Geometry: final body of the model. Coordinates: model frame, mm. A direction names the side the tool comes from. Round coordinates to 2 decimals unless told otherwise and drop trailing zeros. Loops run counter-clockwise (first coordinate to the right, second up) from the corner with the lowest first, then second, coordinate; pieces in that order, holes last. Notation, with made-up numbers: (21.25, -13) - (64.25, -13) arc R22 ccw to (64.25, -3) - close; hole circle Ø1 at (87, -1.5). An arc over 180 degrees is marked (long way). Return JSON: item names as keys, results as strings. Group by question number.
1. Draft query along Z for faces 6 (the face through (1.97, -17.85, -11.57)), 7 (the face through (2, -10, -5)), 8 (the face through (2, -20.5, -7)). Return one class per face: +Z half, -Z half, draft (parallel to the pull), parting line (faces both ways), or undercut.
2. Section B-B on x = 3.2. Return loops of the section in (y, z).
3. First-contact query: pin 1 Ø0.8 at (x, y) = (0.5, -2.5) entering from +Z; pin 2 Ø1 at (x, z) = (3, -10) entering from +Y; pin 3 Ø6 at (y, z) = (-8, -1.5) entering from +X; pin 4 Ø0.8 at (x, y) = (1, -6.5) entering from -Z. Flat tips, straight axial feed; report the tip coordinate or a pass-through.
4. Section D-D on y = -6.5. Return loops of the section in (x, z).
5. Section C-C on z = -7.5. Return loops of the section in (x, y).
6. Material intervals for probe 1 along Y at (x, z) = (2.85, -9.75); probe 2 along Y at (x, z) = (3, -5.5); probe 3 along X at (y, z) = (-2, -3.5), sorted ascending.
7. Section A-A on z = -10.25. Return loops of the section in (x, y), and give its area (3 significant figures).
8. Set-up query: faces 1 (the face through (1, -5, -10)), 2 (the face through (2, -19.2, -3.7)), 3 (the face through (2, -20.1, -10)), 4 (the face through (1, -5, 0)), 5 (the face through (1.6, -5, -5)). Return all of +Z, -Z, +X, -X, +Y, -Y with unobstructed straight access to the full face (end or side cutting, diameter ignored); none if empty.
from build123d import *

# Parameters (mm, degrees)
SKETCH1_W           = 10
SKETCH1_H           = 10
BOSS_EXTRUDE1_DEPTH = 1.6
BOSS_EXTRUDE2_DEPTH = 10
SKETCH3_W           = 4
SKETCH3_H           = 2
BOSS_EXTRUDE3_DEPTH = 2
SKETCH4_W           = 4
SKETCH4_H           = 2
BOSS_EXTRUDE4_DEPTH = 2
BOSS_EXTRUDE5_DEPTH = 4
FILLET2_R           = 1.5


with BuildPart() as part:
    # Sketch1 → Boss-Extrude1 (new body)
    with BuildSketch(Plane(origin=(0, 0, 0), x_dir=(0, 0, -1), z_dir=(1, 0, 0))):
        with Locations((5, -5)):
            Rectangle(SKETCH1_W, SKETCH1_H)
    extrude(amount=BOSS_EXTRUDE1_DEPTH)

    # Sketch2 → Boss-Extrude2 (add)
    with BuildSketch(Plane.XY):
        Polygon((1.2, -12), (0, -12), (0, -10), (1.6, -10), (4, -10), (4, -12), (2.8, -12), align=None)
    extrude(amount=-BOSS_EXTRUDE2_DEPTH)

    # Sketch3 → Boss-Extrude3 (add)
    with BuildSketch(Plane.XY):
        with Locations((2, -11)):
            Rectangle(SKETCH3_W, SKETCH3_H)
    extrude(amount=BOSS_EXTRUDE3_DEPTH)

    # Sketch4 → Boss-Extrude4 (add)
    with BuildSketch(Plane(origin=(0, 0, -10), x_dir=(-1, 0, 0), z_dir=(0, 0, -1))):
        with Locations((-2, -11)):
            Rectangle(SKETCH4_W, SKETCH4_H)
    extrude(amount=BOSS_EXTRUDE4_DEPTH)

    # Sketch5 → Boss-Extrude5 (add)
    with BuildSketch(Plane(origin=(4, 0, 0), x_dir=(0, 0, -1), z_dir=(1, 0, 0))):
        with BuildLine():
            Line((12, -12), (-2, -12))
            Line((-2, -12), (-2, -16.665516671))
            Line((-2, -16.665516671), (-2, -18.3))
            Line((-2, -18.3), (-2, -20.1))
            Line((-2, -20.1), (-2, -22))
            ThreePointArc((-2, -22), (-1.560660172, -23.060660172), (-0.5, -23.5))
            Line((-0.5, -23.5), (10.5, -23.5))
            ThreePointArc((10.5, -23.5), (11.560660172, -23.060660172), (12, -22))
            Line((12, -22), (12, -20.1))
            Line((12, -20.1), (9.118083152, -20.1))
            ThreePointArc((9.118083152, -20.1), (8.689901951, -20.395826074), (8.18, -20.5))
            Line((8.18, -20.5), (5, -20.5))
            ThreePointArc((5, -20.5), (3.7, -19.2), (5, -17.9))
            Line((5, -17.9), (8.18, -17.9))
            ThreePointArc((8.18, -17.9), (8.689901951, -18.004173926), (9.118083152, -18.3))
            Line((9.118083152, -18.3), (12, -18.3))
            Line((12, -18.3), (12, -12))
        make_face()
    extrude(amount=-BOSS_EXTRUDE5_DEPTH)

    # Fillet2
    fillet2_edges = [part.edges().sort_by_distance(p)[0] for p in [
        (2, -18.3, -12),
        (2, -18.3, -9.118083152),
        (2, -20.1, -9.118083152),
        (2, -20.1, -12),
    ]]
    fillet(fillet2_edges, radius=FILLET2_R)


solid = part.part
Taken from the geometry:
{
 "1": {"face 6": "-Z half", "face 7": "draft", "face 8": "undercut"},
 "2": {"outline": "(-23.5, -10.5) arc R1.5 ccw to (-22, -12) - (-21.6, -12) arc R1.5 ccw to (-20.1, -10.5) - (-20.1, -9.62) arc R1.5 ccw to (-20.31, -8.85) arc R1.3 cw to (-20.5, -8.18) - (-20.5, -5) arc R1.3 cw to (-17.9, -5) - (-17.9, -8.18) arc R1.3 cw to (-18.09, -8.85) arc R1.5 ccw to (-18.3, -9.62) - (-18.3, -10.5) arc R1.5 ccw to (-16.8, -12) - (-10, -12) - (-10, 2) - (-22, 2) arc R1.5 ccw to (-23.5, 0.5) - close"},
 "3": {"pin 1": "z = 0", "pin 2": "y = -10", "pin 3": "x = 4", "pin 4": "z = -10"},
 "4": {"outline": "(0, -10) - (1.6, -10) - (1.6, 0) - (0, 0) - close"},
 "5": {"outline": "(0, -23.5) - (4, -23.5) - (4, -20.5) - (0, -20.5) - close; (0, -17.9) - (4, -17.9) - (4, -10) - (1.6, -10) - (1.6, 0) - (0, 0) - close"},
 "6": {"probe 1": "-23.5 to -20.1, -18.3 to -10", "probe 2": "-23.5 to -20.5, -17.9 to -10", "probe 3": "0 to 1.6"},
 "7": {"outline": "(0, -23.5) - (4, -23.5) - (4, -20.1) - (0, -20.1) - close; (0, -18.3) - (4, -18.3) - (4, -10) - (0, -10) - close", "area": "46.8 mm2"},
 "8": {"face 1": "-Z, +X, -X, +Y", "face 2": "+X, -X", "face 3": "-Z, +X, -X", "face 4": "+Z, +X, -X, +Y", "face 5": "+Z, -Z, +X, +Y"}
}
